Autodesk Inventor part; units mm, degrees
ref_plane "YZ Plane" through (0, 0, 0) normal (1, 0, 0) x (0, 1, 0)
ref_plane "XZ Plane" through (0, 0, 0) normal (0, 1, 0) x (-1, 0, 0)
ref_plane "XY Plane" through (0, 0, 0) normal (0, 0, 1) x (1, 0, 0)
sketch "Sketch2" plane through (0, 0, 0) normal (1, 0, 0) x (0, 1, 0)
  line L0 (0, 0) -> (30, 0)
  line L1 (30, 60) -> (30, -60)
  line L2 (30, 60) -> (27, 60)
  line L3 (27, 60) -> (27, -60)
  line L4 (27, -60) -> (30, -60)
  line L5 (27, 60) -> (0, 60)
  line L6 (0, 60) -> (5, 60)
  line L7 (5, 60) -> (5, 54)
  line L8 (5, 54) -> (27, 54)
  line L9 (27, -60) -> (0, -60)
  line L10 (0, -60) -> (5, -60)
  line L11 (5, -60) -> (5, -54)
  line L12 (5, -54) -> (27, -54)
  line L13 (0, 60) -> (0, -60)
  line L14 (27, 0) -> (28, 0)
  line L15 (28, 0) -> (28, -3)
  line L16 (28, -3) -> (27, -3)
  line L17 (28, 0) -> (28, 2)
  line L18 (28, 2) -> (30, 2)
  line L19 (30, 2) -> (28, 0)
  dimension "d12" = 30
  dimension "d13" = 120
  dimension "d14" = 3
  dimension "d15" = 5
  dimension "d16" = 6
  dimension "d17" = 6
  dimension "d26" = 1
  dimension "d27" = 3
  dimension "d28" = 2
revolve "Revolution1" add sketch "Sketch2" angle 360 about axis through (0, 0, 60) along (0, 0, -1) contours L3 L2 L1 L18 L17 L0 | L0 L15 L16 L3 | L17 L18 L19 | L8 L7 L5 L3
fillet "Fillet2" radius 3 1 edges at (0, -30, 60)
thread "Thread3"
chamfer "Chamfer2" distance 0.5 angle 45 1 edges at (0, -5, 60)
fillet "Fillet3" radius 3 1 edges at (0, -27, 54)
chamfer "Chamfer3" distance 0.2 angle 45 1 edges at (0, -28, -3)
properties part number "Plenum"
The model under review builds one solid part; all positions refer to its coordinate system, in mm. Round coordinates to 2 decimals unless told otherwise and drop trailing zeros. Write each loop counter-clockwise with the first axis right and the second up, starting at its lowest first coordinate (ties: lowest second). Pieces come first, ordered by that corner, then holes. Notation, with made-up numbers: (-22, 12.5) -> (21, 12.5) arc R28 ccw to (21, 47.5) -> close; hole circle Ø8 at (16.5, 15.5). An arc over 180 degrees is marked (long way). Use CSV: the item, a comma, the result in double quotes.
Q1. Mouldability with a two-part tool opening along Y and no side actions: class faces 1 (the cylindrical face through (-10.724, 25.865, -1.42)), 2 (the cylindrical face through (-26.36, -5.85, 23.62)), 3 (the flat face through (0, 6, 60)), 4 (the flat face through (6, 0, 54)) as released by +Y, released by -Y, zero draft, split by the parting line, or undercut.
Checks:
face 1,"split by the parting line"
face 2,"undercut"
face 3,"zero draft"
face 4,"undercut"
Q2. Consider section C-C (z = 17.5). Give the boundary of the cut face in (x, y).
Checks:
outline,"circle Ø60 at (0, 0); hole circle Ø54 at (0, 0)"
Q3. For pin 1 Ø2 at (y, z) = (17.5, 29) entering from +X; pin 2 Ø10 at (x, z) = (-2, 42.5) entering from +Y; pin 3 Ø5 at (y, z) = (-21, 44.5) entering from +X; pin 4 Ø8 at (y, z) = (6.5, 35.5) entering from -X, all flat-tipped, find the tip position at first contact; note any pin that passes through.
Checks:
pin 1,"x = 25.05"
pin 2,"y = 30"
pin 3,"x = 23.62"
pin 4,"x = -29.9"
Q4. Consider section A-A (y = 0). Give the boundary of the cut face in (x, z), then the cut area to 3 significant figures.
Checks:
outline,"(-30, 2) -> (-28, 0) -> (-28, -2.8) -> (-27.8, -3) -> (-27, -3) -> (-27, 51) arc R3 cw to (-24, 54) -> (-5, 54) -> (-5, 59.5) -> (-5.5, 60) -> (-27, 60) arc R3 ccw to (-30, 57) -> close; (5, 54) -> (24, 54) arc R3 cw to (27, 51) -> (27, -3) -> (27.8, -3) -> (28, -2.8) -> (28, 0) -> (30, 2) -> (30, 57) arc R3 ccw to (27, 60) -> (5.5, 60) -> (5, 59.5) -> close"
area,"626 mm²"
Q5. To check wall thickness, follow probe 1 along X at (y, z) = (0, 35.5); probe 2 along Z at (x, y) = (-7, -2.5); probe 3 along X at (y, z) = (0, 56.75). State the ranges of each line that lie inside material, in increasing order. Write a range as [from, to].
Checks:
probe 1,"[-30, -27], [27, 30]"
probe 2,"[54, 60]"
probe 3,"[-30, -5], [5, 30]"
